Model file for the job. Use its own axes, mm. Round coordinates to 2 decimals unless told otherwise and drop trailing zeros. Order: outer loops, then holes, each group sorted by start corner. A loop starts at its lowest first (then second) coordinate and runs counter-clockwise, first axis right, second up. Notation, with made-up numbers: (84.5, 3) -> (122.5, 3) arc R28 cw to (122.5, 35) -> close; hole circle Ø5 at (-14.5, -35.75). An arc over 180 degrees is marked (long way). Use CSV: the item, a comma, the result in double quotes.
```python
from build123d import *

# Parameters (mm, degrees)
CROQUIS2_R                   = 40
CROQUIS2_R_2                 = 20
SALIENTE_EXTRUIR1_DEPTH      = 10
SALIENTE_EXTRUIR1_DEPTH_BACK = 10


with BuildPart() as part:
    # Croquis2 → Saliente-Extruir1 (new body, two sides)
    with BuildSketch(Plane(origin=(0, 0, 0), x_dir=(1, 0, 0), z_dir=(0, 1, 0))) as saliente_extruir1_sk:
        with BuildLine():
            ThreePointArc((172.469235199, 66.119242389), (218.184271838, 88.238889892), (205.354467187, 137.376853761))
            ThreePointArc((205.354467187, 137.376853761), (24.626451497, 155.299352148), (-79.722697138, 6.655190531))
            ThreePointArc((-79.722697138, 6.655190531), (-5.078826092, -79.838621766), (79.923379849, -3.500479035))
            ThreePointArc((79.923379849, -3.500479035), (109.764419077, 53.152375878), (172.469235199, 66.119242389))
        make_face()
        Circle(CROQUIS2_R, mode=Mode.SUBTRACT)
        with Locations((181.865334795, 105)):
            Circle(CROQUIS2_R_2, mode=Mode.SUBTRACT)
    extrude(amount=SALIENTE_EXTRUIR1_DEPTH)
    extrude(saliente_extruir1_sk.sketch, amount=-SALIENTE_EXTRUIR1_DEPTH_BACK)


solid = part.part
```
Q1. Cut at B-B (x = 0). Give the cut face in (y, z), plus the area to 3 significant figures.
From the geometry:
outline,"(-10, -141.58) -> (10, -141.58) -> (10, -40) -> (-10, -40) -> close; (-10, 40) -> (10, 40) -> (10, 80) -> (-10, 80) -> close"
area,"2,830 mm²"
Q2. Cut at C-C (y = 0.25). Give the cut face in (x, z), plus the area to 3 significant figures.
From the geometry:
outline,"(-79.72, -6.66) arc R180 ccw to (205.35, -137.38) arc R40 ccw to (172.47, -66.12) arc R75 cw to (79.92, 3.5) arc R80 ccw (long way) to start; hole circle Ø80 at (0, 0); hole circle Ø40 at (181.87, -105)"
area,"38,200 mm²"
Q3. Cut at A-A (z = -105). Give the cut face in (x, y).
From the geometry:
outline,"(-40.2, -10) -> (161.87, -10) -> (161.87, 10) -> (-40.2, 10) -> close; (201.87, -10) -> (221.87, -10) -> (221.87, 10) -> (201.87, 10) -> close"
Q4. Pin check, flat tips, straight feed: pin 1 (8 mm diameter, centred on x = 66.5, y = 0.5, fed in from +Z); pin 2 (10 mm diameter, centred on y = -3, z = 50.5, fed in from +X); pin 3 (3 mm diameter, centred on x = 8.5, y = 3, fed in from +Z). Stop position of each tip, or through.
From the geometry:
pin 1,"stops at z = 49.94"
pin 2,"stops at x = 65.8"
pin 3,"stops at z = 79.69"
Q5. Probe line 1 along Z through (x, y) = (36.5, -3.5); line 2 along Z through (x, y) = (167, -3); line 3 along X through (y, z) = (3.5, -105). List the from-to ranges inside material, lowest first.
From the geometry:
line 1,"z = -160.24 to -16.36, 16.36 to 71.19"
line 2,"z = -158.61 to -118.38, -91.62 to -67.23"
line 3,"x = -40.2 to 161.87, 201.87 to 221.87"
Q6. Cut at D-D (z = -61.5). Give the cut face in (x, y).
From the geometry:
outline,"(-66.25, -10) -> (123.83, -10) -> (123.83, 10) -> (-66.25, 10) -> close"
Q7. Mould opens along Z. For faces 1 (the cylindrical face through (217.855, 0.14, -87.543)), 2 (the flat face through (69, 10, -76)), 3 (the cylindrical face through (-8.67, -0.14, 39.05)) say: +Z half, -Z half, draft (parallel to the pull), parting line (faces both ways), or undercut.
From the geometry:
face 1,"parting line"
face 2,"draft"
face 3,"undercut"
